The model under review builds one solid part; all positions refer to its coordinate system, in mm. Coordinates: 2 decimals unless noted, no trailing zeros. Write each loop counter-clockwise with the first axis right and the second up, starting at its lowest first coordinate (ties: lowest second). Pieces come first, ordered by that corner, then holes. Notation, with made-up numbers: (69, -15.5) - (78, -15.5) arc R10 cw to (78, -11.5) - close; hole circle Ø11 at (-13, 42.5). An arc over 180 degrees is marked (long way). Return JSON: item names as keys, results as strings. Group by question number.
(1) To check wall thickness, follow L1, parallel to Y at x = 210.5, z = 14; L2, parallel to Z at x = 211, y = 22.25 (3 decimals); L3, parallel to X at y = 15.5, z = 12 (3 decimals). State the ranges of each line that lie inside material, in increasing order. Write a range as from..to.
(2) We need section A-A on x = 236.5. State the section outline as (y, z) points (3 decimals), then the cut area to 3 significant figures.
(3) For pin 1 Ø7.5 at (x, y) = (283.5, 26) entering from +Z (3 decimals); pin 2 Ø4 at (y, z) = (32.5, 7.5) entering from +X; pin 3 Ø9.5 at (x, z) = (-62, 6.5) entering from +Y, all flat-tipped, find the tip position at first contact; note any pin that passes through.
(4) We need section B-B on z = 6. State the section outline as (x, y) points (3 decimals).
Autodesk Inventor part; units mm, degrees
ref_plane "YZ Plane" through (0, 0, 0) normal (1, 0, 0) x (0, 1, 0)
ref_plane "XZ Plane" through (0, 0, 0) normal (0, 1, 0) x (-1, 0, 0)
ref_plane "XY Plane" through (0, 0, 0) normal (0, 0, 1) x (1, 0, 0)
sketch "Sketch1" plane through (0, 0, 0) normal (0, 0, 1) x (1, 0, 0)
  line L0 (-47.625, 38.3646) -> (-47.625, 30.4271)
  line L1 (-47.625, 30.4271) -> (-66.675, 30.4271)
  line L2 (-66.675, 30.4271) -> (-66.675, 20.9021)
  line L3 (-66.675, 20.9021) -> (-47.625, 20.9021)
  line L4 (-47.625, 20.9021) -> (-47.625, 12.9646)
  line L5 (-47.625, 38.3646) -> (185.7375, 38.3646)
  line L6 (185.7375, 38.3646) -> (185.7375, 12.9646)
  line L7 (185.7375, 12.9646) -> (-47.625, 12.9646)
  line L8 (-47.625, 12.9646) -> (-47.625, 38.3646)
  line L9 (-47.625, 20.9021) -> (-66.675, 20.9021)
  line L10 (-66.675, 20.9021) -> (-66.675, 30.4271)
  line L11 (-66.675, 30.4271) -> (-47.625, 30.4271)
  line L12 (-47.625, 30.4271) -> (-47.625, 20.9021)
  point P0 (0, 0)
  dimension "d0" = 7.9375
  dimension "d1" = 19.05
  dimension "d2" = 9.525
  dimension "d3" = 7.9375
  dimension "d4" = 25.4
  dimension "d6" = 252.4125
extrude "Extrusion1" add sketch "Sketch1" along normal blind 19.05
mirror "Mirror1" about plane through (185.7375, 12.9646, 0) normal (1, 0, 0) of "Extrusion1"
sketch "Sketch2" plane through (0, 0, 19.05) normal (0, 0, 1) x (1, 0, 0)
  line L0 (-66.675, 30.4271) -> (-66.675, 20.9021)
  line L1 (-47.625, 12.9646) -> (419.1, 12.9646)
  line L2 (438.15, 30.4271) -> (438.15, 20.9021)
  line L3 (-47.625, 38.3646) -> (419.1, 38.3646)
  line L4 (-42.8625, 30.4271) -> (414.3375, 30.4271)
  line L5 (414.3375, 30.4271) -> (414.3375, 20.9021)
  line L6 (414.3375, 20.9021) -> (-42.8625, 20.9021)
  line L7 (-42.8625, 20.9021) -> (-42.8625, 30.4271)
  point P0 (0, 0)
  dimension "d10" = 7.9375
  dimension "d11" = 7.9375
  dimension "d12" = 9.525
  dimension "d13" = 23.8125
  dimension "d14" = 23.8125
extrude "Extrusion2" cut sketch "Sketch2" against normal blind 9.525
equation "\"d11\" = d10"
properties part number "top_cover_side" material "Wood (Birch)"
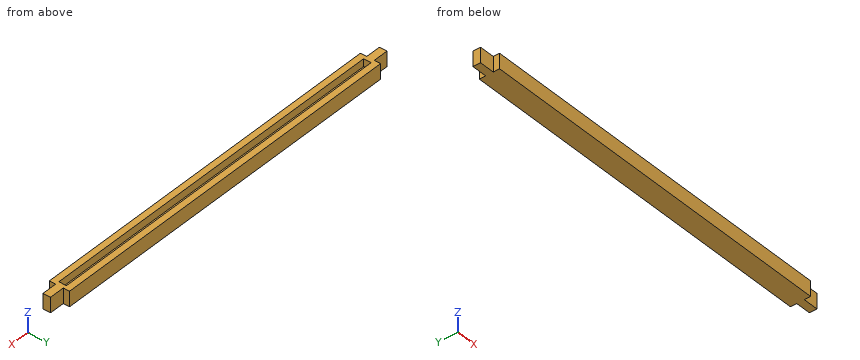
Ans:
{
 "1": {"L1": "12.96..20.9, 30.43..38.36", "L2": "0..9.525", "L3": "-47.625..419.1"},
 "2": {"outline": "(12.965, 0) - (38.365, 0) - (38.365, 19.05) - (30.427, 19.05) - (30.427, 9.525) - (20.902, 9.525) - (20.902, 19.05) - (12.965, 19.05) - close", "area": "393 mm²"},
 "3": {"pin 1": "z = 9.525", "pin 2": "x = 419.1", "pin 3": "y = 30.43"},
 "4": {"outline": "(-66.675, 20.902) - (-47.625, 20.902) - (-47.625, 12.965) - (419.1, 12.965) - (419.1, 20.902) - (438.15, 20.902) - (438.15, 30.427) - (419.1, 30.427) - (419.1, 38.365) - (-47.625, 38.365) - (-47.625, 30.427) - (-66.675, 30.427) - close"}
}
